Check sheet for the modelled part. Datum: model origin and axes. Units: mm. Face numbers are marked on the shaded views. Round coordinates to 2 decimals unless told otherwise and drop trailing zeros. Write each loop counter-clockwise with the first axis right and the second up, starting at its lowest first coordinate (ties: lowest second). Pieces come first, ordered by that corner, then holes. Notation, with made-up numbers: M 30.5,56 L 71.5,56 A20 ccw 71.5,62 Z; hole C -22,-39 d2. An arc over 180 degrees is marked long. Answer in a Markdown table with one row per item.
```python
from build123d import *

# Parameters (mm, degrees)
SKETCH_1_R          = 17.5
EXTRUDE_1_DEPTH     = 2
CUT_EXTRUDE_2_REACH = 26.829
SKETCH_1_4_W        = 26.2
SKETCH_1_4_H        = 2.6
SKETCH_1_4_R        = 1.1
SKETCH_1_5_R        = 2.3
SKETCH_1_5_R_2      = 1.45
EXTRUDE_2_DEPTH     = 4
SKETCH_1_6_R        = 1.75
SKETCH_1_6_R_2      = 0.95
EXTRUDE_3_DEPTH     = 11


with BuildPart() as part:
    # 草图1 → 凸台-拉伸1 (new body)
    with BuildSketch(Plane(origin=(0, 0, 0), x_dir=(1, 0, 0), z_dir=(0, 1, 0))):
        with Locations(Location((-4.53e-07, -7.66e-07, 0), (0, 0, 270))):
            Circle(SKETCH_1_R)
    extrude(amount=EXTRUDE_1_DEPTH)

    # 草图1<4> → 切除-拉伸2 (cut, up to next)
    with BuildSketch(Plane(origin=(0, 0, 0), x_dir=(1, 0, 0), z_dir=(0, 1, 0)), mode=Mode.PRIVATE) as cut_extrude_2_sk1:
        with Locations((-4.53e-07, 7.806744123)):
            Rectangle(SKETCH_1_4_W, SKETCH_1_4_H)
    cut_extrude_2_tool1 = extrude(cut_extrude_2_sk1.sketch, amount=CUT_EXTRUDE_2_REACH, mode=Mode.PRIVATE) & part.part
    # 草图1<4> → 切除-拉伸2 (cut, up to next)
    with BuildSketch(Plane(origin=(0, 0, 0), x_dir=(1, 0, 0), z_dir=(0, 1, 0)), mode=Mode.PRIVATE) as cut_extrude_2_sk2:
        with Locations(Location((-6.499999337, -11.258330632, 0), (0, 0, 270))):
            Circle(SKETCH_1_4_R)
    cut_extrude_2_tool2 = extrude(cut_extrude_2_sk2.sketch, amount=CUT_EXTRUDE_2_REACH, mode=Mode.PRIVATE) & part.part
    # 草图1<4> → 切除-拉伸2 (cut, up to next)
    with BuildSketch(Plane(origin=(0, 0, 0), x_dir=(1, 0, 0), z_dir=(0, 1, 0)), mode=Mode.PRIVATE) as cut_extrude_2_sk3:
        with Locations(Location((13, 7.66e-07, 0), (0, 0, 270))):
            Circle(SKETCH_1_4_R)
    cut_extrude_2_tool3 = extrude(cut_extrude_2_sk3.sketch, amount=CUT_EXTRUDE_2_REACH, mode=Mode.PRIVATE) & part.part
    # 草图1<4> → 切除-拉伸2 (cut, up to next)
    with BuildSketch(Plane(origin=(0, 0, 0), x_dir=(1, 0, 0), z_dir=(0, 1, 0)), mode=Mode.PRIVATE) as cut_extrude_2_sk4:
        with Locations(Location((-6.500000663, 11.258329866, 0), (0, 0, 270))):
            Circle(SKETCH_1_4_R)
    cut_extrude_2_tool4 = extrude(cut_extrude_2_sk4.sketch, amount=CUT_EXTRUDE_2_REACH, mode=Mode.PRIVATE) & part.part
    add(cut_extrude_2_tool1.solids().sort_by_distance((0, 0, -7.806744))[0], mode=Mode.SUBTRACT)
    add(cut_extrude_2_tool2.solids().sort_by_distance((-6.499999, 0, 11.258331))[0], mode=Mode.SUBTRACT)
    add(cut_extrude_2_tool3.solids().sort_by_distance((13, 0, -1e-06))[0], mode=Mode.SUBTRACT)
    add(cut_extrude_2_tool4.solids().sort_by_distance((-6.500001, 0, -11.25833))[0], mode=Mode.SUBTRACT)

    # 草图1<5> → 凸台-拉伸2 (add)
    # profile 1 of 2: a face of its own
    with BuildSketch(Plane(origin=(0, 0, 0), x_dir=(1, 0, 0), z_dir=(0, 1, 0))):
        with Locations(Location((-10, -3.793255877, 0), (0, 0, 270))):
            Circle(SKETCH_1_5_R)
        with Locations(Location((-10, -3.793255877, 0), (0, 0, 270))):
            Circle(SKETCH_1_5_R_2, mode=Mode.SUBTRACT)
    # profile 2 of 2: a face of its own
    with BuildSketch(Plane(origin=(0, 0, 0), x_dir=(1, 0, 0), z_dir=(0, 1, 0))):
        with Locations(Location((10, -3.793255877, 0), (0, 0, 270))):
            Circle(SKETCH_1_5_R)
        with Locations(Location((10, -3.793255877, 0), (0, 0, 270))):
            Circle(SKETCH_1_5_R_2, mode=Mode.SUBTRACT)
    extrude(amount=EXTRUDE_2_DEPTH)

    # 草图1<6> → 凸台-拉伸3 (add)
    # profile 1 of 2: a face of its own
    with BuildSketch(Plane(origin=(0, 0, 0), x_dir=(1, 0, 0), z_dir=(0, 1, 0))):
        with Locations(Location((0, 12, 0), (0, 0, 270))):
            Circle(SKETCH_1_6_R)
        with Locations(Location((0, 12, 0), (0, 0, 270))):
            Circle(SKETCH_1_6_R_2, mode=Mode.SUBTRACT)
    # profile 2 of 2: a face of its own
    with BuildSketch(Plane(origin=(0, 0, 0), x_dir=(1, 0, 0), z_dir=(0, 1, 0))):
        with Locations(Location((0.002, -12, 0), (0, 0, 270))):
            Circle(SKETCH_1_6_R)
        with Locations(Location((0.002, -12, 0), (0, 0, 270))):
            Circle(SKETCH_1_6_R_2, mode=Mode.SUBTRACT)
    extrude(amount=EXTRUDE_3_DEPTH)


solid = part.part
```
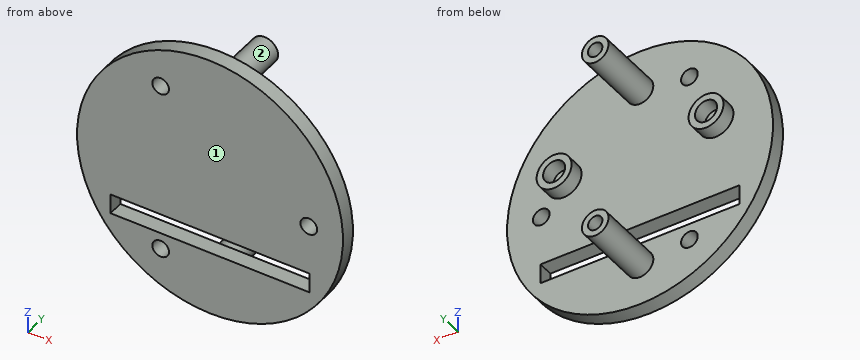
1. Section check D-D, the plane y = 5.5. Record the cut outline in (x, z).
Found:
| item | result |
|---|---|
| outline | C 0,-12 d3.5; C 0,12 d3.5; hole C 0,-12 d1.9; hole C 0,12 d1.9 |
2. Go/stop test with flat-tipped pins: pin 1 (2 mm diameter, centred on x = 1, y = 1.5, fed in from -Z); pin 2 (1.5 mm diameter, centred on y = 6, z = 12, fed in from +X); pin 3 (2 mm diameter, centred on x = 13, z = 0, fed in from -Y); pin 4 (5 mm diameter, centred on x = 0.5, y = 9, fed in from +Z). Record where each tip stops, or that it passes through.
Found:
| item | result |
|---|---|
| pin 1 | stops at z = -17.5 |
| pin 2 | stops at x = 1.75 |
| pin 3 | passes through |
| pin 4 | stops at z = 13.75 |
3. Draft check along Z on the marked faces 1 and 2. Enter one of: +Z half, -Z half, draft (parallel to the pull), parting line (faces both ways), or undercut.
Found:
| item | result |
|---|---|
| face 1 | draft |
| face 2 | undercut |
4. Scan lines: L1, parallel to Z at x = 0, y = 7; L2, parallel to X at y = 1.3, z = 0; L3, parallel to Y at x = -14.5, z = -4.5. Record each from-to range of solid material in increasing order.
Found:
| item | result |
|---|---|
| L1 | z = -13.75 to -12.95, -11.05 to -10.25, 10.25 to 11.05, 12.95 to 13.75 |
| L2 | x = -17.5 to 11.9, 14.1 to 17.5 |
| L3 | y = 0 to 2 |
5. Section check A-A, the plane y = 1.5. Record the cut outline in (x, z), and give its area (3 significant figures).
Found:
| item | result |
|---|---|
| outline | C 0,0 d35; hole M -13.1,-9.11 L 13.1,-9.11 L 13.1,-6.51 L -13.1,-6.51 Z; hole C -6.5,-11.26 d2.2; hole C -6.5,11.26 d2.2; hole C 13,0 d2.2 |
| area | 883 mm2 |
6. Section check C-C, the plane x = 3.5. Record the cut outline in (y, z), and give its area (3 significant figures).
Found:
| item | result |
|---|---|
| outline | M 0,-17.15 L 2,-17.15 L 2,-9.11 L 0,-9.11 Z; M 0,-6.51 L 2,-6.51 L 2,17.15 L 0,17.15 Z |
| area | 63.4 mm2 |
7. Section check B-B, the plane z = 0. Record the cut outline in (x, y).
Found:
| item | result |
|---|---|
| outline | M -17.5,0 L 11.9,0 L 11.9,2 L -17.5,2 Z; M 14.1,0 L 17.5,0 L 17.5,2 L 14.1,2 Z |
